Check sheet for the modelled part. Datum: model origin and axes. Units: mm. A direction names the side the tool comes from. Give positions to 0.01 mm unless a question says otherwise; leave off trailing zeros. Order: outer loops, then holes, each group sorted by start corner. A loop starts at its lowest first (then second) coordinate and runs counter-clockwise, first axis right, second up.
Item 1: Material ranges on line 1 along Z through (x, y) = (3.81, -0.7); line 2 along Z through (x, y) = (21.59, -0.6); line 3 along Z through (x, y) = (24.5, -1.1), recorded low to high.
Item 2: Sectioned sample at B-B on y = -2.8. Record the boundary of the cut face in (x, z).
Item 3: Gauge pin test, flat ends, axial feed: P1, Ø1.5, axis at x = 14.5, z = 2, coming from the -Y side; P2, Ø1.6, axis at x = 1.5, y = -2.5, coming from the +Z side. Record the tip position at first contact, or that the pin passes through.
Item 4: Sectioned sample at A-A on x = 34.29. Count the separate pieces of the cut face and the enclosed holes in it, and give its area (3 significant figures).
Item 5: Access from +Z, -Z, +X, -X, +Y, -Y to the whole of each face (thin tool, end or side, straight path). Record for faces 4 (the flat face through (5, -3, 9)), 5 (the cylindrical face through (35.13, -0.77, 13.62)), 6 (the flat face through (32.34, -3, 9)).
Item 6: Release check for a two-part mould opening along Z. For faces 1 (the flat face through (18, 0, 9)), 2 (the cylindrical face through (15.6, -0.8, 1.3)), 3 (the flat face through (31, -3, 7.39)) record: released by +Z, released by -Z, zero draft, split by the parting line, or undercut.
Item 7: Sectioned sample at C-C on x = 1.27. Record the boundary of the cut face in (y, z).
from build123d import *

# Parameters (mm, degrees)
F0_W     = 35.56
F0_H     = 17.78
F0_R     = 0.912
F1_DEPTH = 1.57
F3_DEPTH = 2.5
F4_R     = 0.5
F6_DEPTH = 2.5
F7_R     = 0.5


with BuildPart() as f1:
    # F0 (on Front) → F1 (new body)
    with BuildSketch(Plane.XZ):
        with Locations((17.78, 8.89)):
            Rectangle(F0_W, F0_H)
        with Locations((1.27, 1.27)):
            Circle(F0_R, mode=Mode.SUBTRACT)
        with Locations((3.81, 1.27)):
            Circle(F0_R, mode=Mode.SUBTRACT)
        with Locations((6.35, 1.27)):
            Circle(F0_R, mode=Mode.SUBTRACT)
        with Locations((8.89, 1.27)):
            Circle(F0_R, mode=Mode.SUBTRACT)
        with Locations((11.43, 1.27)):
            Circle(F0_R, mode=Mode.SUBTRACT)
        with Locations((13.97, 1.27)):
            Circle(F0_R, mode=Mode.SUBTRACT)
        with Locations((16.51, 1.27)):
            Circle(F0_R, mode=Mode.SUBTRACT)
        with Locations((19.05, 1.27)):
            Circle(F0_R, mode=Mode.SUBTRACT)
        with Locations((21.59, 1.27)):
            Circle(F0_R, mode=Mode.SUBTRACT)
        with Locations((24.13, 1.27)):
            Circle(F0_R, mode=Mode.SUBTRACT)
        with Locations((26.67, 1.27)):
            Circle(F0_R, mode=Mode.SUBTRACT)
        with Locations((29.21, 1.27)):
            Circle(F0_R, mode=Mode.SUBTRACT)
        with Locations((31.75, 1.27)):
            Circle(F0_R, mode=Mode.SUBTRACT)
        with Locations((34.29, 1.27)):
            Circle(F0_R, mode=Mode.SUBTRACT)
        with Locations((34.29, 3.81)):
            Circle(F0_R, mode=Mode.SUBTRACT)
        with Locations((34.29, 6.35)):
            Circle(F0_R, mode=Mode.SUBTRACT)
        with BuildLine():
            ThreePointArc((33.378, 8.89), (34.29, 9.802), (35.202, 8.89))
            ThreePointArc((35.202, 8.89), (34.29, 7.978), (33.378, 8.89))
        make_face(mode=Mode.SUBTRACT)
        with Locations((3.81, 13.97)):
            Circle(F0_R, mode=Mode.SUBTRACT)
        with Locations((8.89, 13.97)):
            Circle(F0_R, mode=Mode.SUBTRACT)
        with Locations((1.27, 16.51)):
            Circle(F0_R, mode=Mode.SUBTRACT)
        with Locations((3.81, 16.51)):
            Circle(F0_R, mode=Mode.SUBTRACT)
        with Locations((6.35, 16.51)):
            Circle(F0_R, mode=Mode.SUBTRACT)
        with Locations((8.89, 16.51)):
            Circle(F0_R, mode=Mode.SUBTRACT)
        with Locations((11.43, 16.51)):
            Circle(F0_R, mode=Mode.SUBTRACT)
        with Locations((13.97, 16.51)):
            Circle(F0_R, mode=Mode.SUBTRACT)
        with Locations((16.51, 16.51)):
            Circle(F0_R, mode=Mode.SUBTRACT)
        with Locations((34.29, 11.43)):
            Circle(F0_R, mode=Mode.SUBTRACT)
        with Locations((19.05, 16.51)):
            Circle(F0_R, mode=Mode.SUBTRACT)
        with Locations((21.59, 16.51)):
            Circle(F0_R, mode=Mode.SUBTRACT)
        with Locations((24.13, 16.51)):
            Circle(F0_R, mode=Mode.SUBTRACT)
        with Locations((34.29, 13.97)):
            Circle(F0_R, mode=Mode.SUBTRACT)
        with Locations((26.67, 16.51)):
            Circle(F0_R, mode=Mode.SUBTRACT)
        with Locations((29.21, 16.51)):
            Circle(F0_R, mode=Mode.SUBTRACT)
        with Locations((31.75, 16.51)):
            Circle(F0_R, mode=Mode.SUBTRACT)
        with Locations((34.29, 16.51)):
            Circle(F0_R, mode=Mode.SUBTRACT)
    extrude(amount=F1_DEPTH)

    # F2 (on face) → F3 (join)
    with BuildSketch(Plane.XZ.offset(1.57)):
        Polygon((5, 12.64), (0, 12.64), (0, 8.89), (0, 5.14), (5, 5.14), (5, 8.89), align=None)
    extrude(amount=F3_DEPTH)

    # F4
    f4_edges = [f1.edges().sort_by_distance(p)[0] for p in [
        (2.5, -4.07, 5.14),
        (2.5, -4.07, 12.64),
        (5, -4.07, 8.89),
    ]]
    fillet(f4_edges, radius=F4_R)

    # F5 (on face) → F6 (join)
    with BuildSketch(Plane.XZ.offset(1.57)):
        Polygon((31.24, 8.89), (30.14, 8.89), (30.14, 7.39), (31.24, 7.39), (32.34, 7.39), (32.34, 8.89), align=None)
        Polygon((30.14, 10.39), (30.14, 8.89), (31.24, 8.89), (32.34, 8.89), (32.34, 10.39), (31.24, 10.39), align=None)
    extrude(amount=F6_DEPTH)

    # F7
    f7_edges = [f1.edges().sort_by_distance(p)[0] for p in [
        (30.14, -2.82, 7.39),
        (32.34, -2.82, 7.39),
        (30.14, -2.82, 10.39),
        (32.34, -2.82, 10.39),
    ]]
    fillet(f7_edges, radius=F7_R)


solid = f1.part
Report:
1. line 1: z = 0 to 0.36, 2.18 to 13.06, 14.88 to 15.6, 17.42 to 17.78
1. line 2: z = 0 to 0.36, 2.18 to 15.6, 17.42 to 17.78
1. line 3: z = 0 to 0.44, 2.1 to 15.68, 17.34 to 17.78
2. outline: (0, 5.14) - (5, 5.14) - (5, 12.64) - (0, 12.64) - close; (30.14, 7.89) arc R0.5 ccw to (30.64, 7.39) - (31.84, 7.39) arc R0.5 ccw to (32.34, 7.89) - (32.34, 9.89) arc R0.5 ccw to (31.84, 10.39) - (30.64, 10.39) arc R0.5 ccw to (30.14, 9.89) - close
3. P1: stops at y = -1.57
3. P2: stops at z = 12.64
4. separate pieces: 8
4. enclosed holes: 0
4. area: 7.87 mm2
5. face 4: +Z, -Z, -Y
5. face 5: +Y, -Y
5. face 6: +Z, -Z, +X, -Y
6. face 1: zero draft
6. face 2: undercut
6. face 3: released by -Z
7. outline: (-4.07, 5.64) arc R0.5 ccw to (-3.57, 5.14) - (-1.57, 5.14) - (-1.57, 2.18) - (0, 2.18) - (0, 15.6) - (-1.57, 15.6) - (-1.57, 12.64) - (-3.57, 12.64) arc R0.5 ccw to (-4.07, 12.14) - close; (-1.57, 0) - (0, 0) - (0, 0.36) - (-1.57, 0.36) - close; (-1.57, 17.42) - (0, 17.42) - (0, 17.78) - (-1.57, 17.78) - close
